Could you check a few things on this model? Use its own coordinates, in mm. A direction names the side the tool comes from. Round coordinates to 2 decimals unless told otherwise and drop trailing zeros. Write each loop counter-clockwise with the first axis right and the second up, starting at its lowest first coordinate (ties: lowest second). Pieces come first, ordered by that corner, then holes.
```python
from build123d import *

# Parameters (mm, degrees)
F0_W     = 6
F0_H     = 0.1
F0_H_2   = 1
F0_W_2   = 2
F0_W_3   = 1
F2_DEPTH = 10
F3_DEPTH = 10
F4_DEPTH = 15


with BuildPart() as f1:
    # F0 (on Front) → F1 (revolve)
    with BuildSketch(Plane.XZ):
        with Locations((-22, 1.05)):
            Rectangle(F0_W, F0_H)
        with Locations((-22, 0.5)):
            Rectangle(F0_W, F0_H_2)
        with Locations((-12, 0.5)):
            Rectangle(F0_W_2, F0_H_2)
        with Locations((-12, 1.05)):
            Rectangle(F0_W_2, F0_H)
        with Locations((-10, 0.5)):
            Rectangle(F0_W_2, F0_H_2)
        with Locations((-8, 0.5)):
            Rectangle(F0_W_2, F0_H_2)
        with Locations((-8, 1.05)):
            Rectangle(F0_W_2, F0_H)
        with Locations((-6, 0.5)):
            Rectangle(F0_W_2, F0_H_2)
        with Locations((-4, 0.5)):
            Rectangle(F0_W_2, F0_H_2)
        with Locations((-4, 1.05)):
            Rectangle(F0_W_2, F0_H)
        with Locations((-2, 0.5)):
            Rectangle(F0_W_2, F0_H_2)
        with Locations((-0.5, 0.5)):
            Rectangle(F0_W_3, F0_H_2)
        with Locations((-0.5, 1.05)):
            Rectangle(F0_W_3, F0_H)
        with Locations((-14, 0.5)):
            Rectangle(F0_W_2, F0_H_2)
        with Locations((-16, 0.5)):
            Rectangle(F0_W_2, F0_H_2)
        with Locations((-16, 1.05)):
            Rectangle(F0_W_2, F0_H)
        with Locations((-18, 0.5)):
            Rectangle(F0_W_2, F0_H_2)
    revolve(axis=Axis((-12.5, 0, 0), (-1, 0, 0)))

    # F2 (add): a face of the model
    f2_faces = [f1.faces().sort_by_distance(p)[0] for p in [
        (-25, 0, 0),
    ]]
    extrude(f2_faces, amount=F2_DEPTH)

    # F3 (add): a face of the model
    f3_faces = [f1.faces().sort_by_distance(p)[0] for p in [
        (-35, 0, 0),
    ]]
    extrude(f3_faces, amount=F3_DEPTH)

    # F4 (add): a face of the model
    f4_faces = [f1.faces().sort_by_distance(p)[0] for p in [
        (-45, 0, 0),
    ]]
    extrude(f4_faces, amount=F4_DEPTH)


solid = f1.part
```
Q1. We'd pull the mould along X, two halves only. Please class faces 1 (the flat face through (0, 0, 0)), 2 (the cylindrical face through (-15.99, 0.33, 1.05)), 3 (the cylindrical face through (-18, -1, 0)), 4 (the flat face through (-60, 0, 0)): pulls with the +X half, pulls with the -X half, needs draft (parallel to the pull), parting line crosses it, or undercut.
Q2. Imagine slicing it at A-A, the plane x = -41. Write out the boundary of the cut face in (y, z).
Q3. If I drill on L1, parallel to X at y = 1, z = -0.25; L2, parallel to Z at x = -37, y = 0.05; L3, parallel to Y at x = -13.5, z = 0.15, over which ranges is the centre line in solid material (lowest first)?
Q4. On a 3-axis mill with a long thin cutter (end or side, diameter ignored), from which of +Z, -Z, +X, -X, +Y, -Y can I reach the whole of each face in a straight line? I mean faces 5 (the cylindrical face through (-6, -1, 0)), 6 (the cylindrical face through (-0.49, 0.33, 1.05)). Say none if no direction works.
Results found:
1. face 1: pulls with the +X half
1. face 2: needs draft
1. face 3: undercut
1. face 4: pulls with the -X half
2. outline: circle Ø2.2 at (0, 0)
3. L1: x = -60 to -19, -17 to -15, -13 to -11, -9 to -7, -5 to -3, -1 to 0
3. L2: z = -1.1 to 1.1
3. L3: y = -0.99 to 0.99
4. face 5: none
4. face 6: +X, -X
